Could you check a few things on this model? Use its own coordinates, in mm. A direction names the side the tool comes from. Give positions to 0.01 mm unless a question says otherwise; leave off trailing zeros. Order: outer loops, then holes, each group sorted by start corner. A loop starts at its lowest first (then second) coordinate and runs counter-clockwise, first axis right, second up. Notation, with made-up numbers: M -13,5.25 L 20,5.25 A7 ccw 20,17.25 Z; hole C -29,-28.75 d3. An arc over 180 degrees is marked long. Use a Markdown table: item, result. Add a question column.
Item 1: For faces 4 (the face through (-60.64, 61.395, 6.439)), 5 (the face through (32, 2, 12.7)), which set-ups out of +Z, -Z, +X, -X, +Y, -Y let a thin tool reach every point of the face, with its end or its side?
Item 2: Suppose I cut it at A-A on x = 0. Write out the boundary of the cut face in (y, z).
Item 3: Suppose I cut it at B-B on z = 8. Count the separate pieces of the cut face and the enclosed holes in it, plus the area to 3 significant figures.
Item 4: If I drill on L1, parallel to Y at x = 0, z = 6; L2, parallel to Y at x = -35, z = 5.5; L3, parallel to X at y = -47.5, z = 10, over which ranges is the centre line in solid material (lowest first)? Write a range as from..to.
Item 5: I'm going to push flat-ended pins straight in: pin 1 Ø1.5 at (y, z) = (-19, 1.5) entering from -X; pin 2 Ø1.5 at (y, z) = (-116, 10) entering from +X; pin 3 Ø1.5 at (x, z) = (-111, 1.5) entering from +Y. Where does each tip first touch, or does it pass through?
Item 6: If we mould it in two halves opening along Y, with no side actions, what happens to faces 1 (the face through (-125.41, -86.59, 6.26)), 2 (the face through (135.976, 42.876, 6.261)), 3 (the face through (-25.249, 140.333, 6.261))? For each: released by +Y, released by -Y, zero draft, split by the parting line, or undercut.
from build123d import *

# Parameters (mm, degrees)
F0_R     = 25.4
F1_DEPTH = 12.7
F3_DEPTH = 25.4


with BuildPart() as f1:
    # F0 (on Top) → F1 (new body)
    with BuildSketch(Plane.XY):
        with BuildLine():
            ThreePointArc((152.210637, -7.594865), (152.352652, -3.798613), (152.4, 0))
            ThreePointArc((152.4, 0), (152.380736, 2.423103), (152.322947, 4.845593))
            ThreePointArc((152.322947, 4.845593), (141.912408, 13.707712), (150.434272, 24.398564))
            ThreePointArc((150.434272, 24.398564), (149.313035, 30.518479), (147.942937, 36.587529))
            ThreePointArc((147.942937, 36.587529), (135.909535, 43.077036), (142.007699, 55.313412))
            ThreePointArc((142.007699, 55.313412), (139.631639, 61.063618), (137.022854, 66.712049))
            ThreePointArc((137.022854, 66.712049), (123.898547, 70.542066), (127.30343, 83.783034))
            ThreePointArc((127.30343, 83.783034), (123.777584, 88.909334), (120.045438, 93.887448))
            ThreePointArc((120.045438, 93.887448), (106.410408, 94.888661), (106.971492, 108.548883))
            ThreePointArc((106.971492, 108.548883), (102.451727, 112.824659), (97.761205, 116.912389))
            ThreePointArc((97.761205, 116.912389), (84.218213, 115.040539), (81.910694, 128.51614))
            ThreePointArc((81.910694, 128.51614), (76.596814, 131.752374), (71.155269, 134.769016))
            ThreePointArc((71.155269, 134.769016), (58.303006, 130.10685), (53.228892, 142.802119))
            ThreePointArc((53.228892, 142.802119), (47.355806, 144.855748), (41.403792, 146.667945))
            ThreePointArc((41.403792, 146.667945), (29.810413, 139.421563), (22.194015, 150.775282))
            ThreePointArc((22.194015, 150.775282), (16.021353, 151.555522), (9.821987, 152.083163))
            ThreePointArc((9.821987, 152.083163), (0, 142.572904), (-9.821987, 152.083163))
            ThreePointArc((-9.821987, 152.083163), (-13.282535, 151.820072), (-16.736195, 151.478249))
            ThreePointArc((-16.736195, 151.478249), (-16.661745, 150.783242), (-16.636886, 150.084702))
            ThreePointArc((-16.636886, 150.084702), (-25.44977, 140.310082), (-36.081733, 148.067108))
            ThreePointArc((-36.081733, 148.067108), (-42.095292, 146.470974), (-48.038691, 144.630717))
            ThreePointArc((-48.038691, 144.630717), (-47.5856, 142.959149), (-47.43299, 141.233999))
            ThreePointArc((-47.43299, 141.233999), (-55.223917, 131.620163), (-66.243396, 137.250036))
            ThreePointArc((-66.243396, 137.250036), (-71.790301, 134.431814), (-77.217553, 131.389533))
            ThreePointArc((-77.217553, 131.389533), (-76.085391, 128.872443), (-75.697812, 126.139803))
            ThreePointArc((-75.697812, 126.139803), (-82.489349, 116.793296), (-93.476655, 120.365589))
            ThreePointArc((-93.476655, 120.365589), (-98.311696, 116.449862), (-102.98288, 112.340048))
            ThreePointArc((-102.98288, 112.340048), (-100.909017, 109.179225), (-100.181858, 105.469379))
            ThreePointArc((-100.181858, 105.469379), (-106.007645, 96.493782), (-116.577616, 98.160172))
            ThreePointArc((-116.577616, 98.160172), (-120.487052, 93.320043), (-124.19567, 88.324377))
            ThreePointArc((-124.19567, 88.324377), (-120.970356, 84.782436), (-119.802768, 80.136498))
            ThreePointArc((-119.802768, 80.136498), (-124.707149, 71.631282), (-134.525062, 71.615415))
            ThreePointArc((-134.525062, 71.615415), (-137.336068, 66.064849), (-139.918176, 60.404173))
            ThreePointArc((-139.918176, 60.404173), (-135.39715, 56.791586), (-133.693165, 51.261044))
            ThreePointArc((-133.693165, 51.261044), (-137.730696, 43.320467), (-146.525595, 41.904774))
            ThreePointArc((-146.525595, 41.904774), (-148.113906, 35.889145), (-149.455356, 29.813698))
            ThreePointArc((-149.455356, 29.813698), (-143.569406, 26.473362), (-141.239, 20.119508))
            ThreePointArc((-141.239, 20.119508), (-144.473844, 12.83157), (-152.048709, 10.341661))
            ThreePointArc((-152.048709, 10.341661), (-152.344113, 4.126898), (-152.385603, -2.094742))
            ThreePointArc((-152.385603, -2.094742), (-145.146605, -4.804697), (-142.106697, -11.911447))
            ThreePointArc((-142.106697, -11.911447), (-144.611911, -18.465977), (-150.850248, -21.678624))
            ThreePointArc((-150.850248, -21.678624), (-149.839684, -27.817785), (-148.579381, -33.910582))
            ThreePointArc((-148.579381, -33.910582), (-140.082526, -35.634948), (-136.257897, -43.415835))
            ThreePointArc((-136.257897, -43.415835), (-138.114625, -49.164318), (-142.98319, -52.740568))
            ThreePointArc((-142.98319, -52.740568), (-140.711332, -58.532735), (-138.20495, -64.227345))
            ThreePointArc((-138.20495, -64.227345), (-128.627028, -64.632158), (-123.951157, -73.000952))
            ThreePointArc((-123.951157, -73.000952), (-125.24773, -77.87968), (-128.795312, -81.471023))
            ThreePointArc((-128.795312, -81.471023), (-125.362592, -86.660144), (-121.72093, -91.704827))
            ThreePointArc((-121.72093, -91.704827), (-111.314719, -90.494981), (-105.730518, -99.358934))
            ThreePointArc((-105.730518, -99.358934), (-106.561474, -103.31384), (-108.913814, -106.599911))
            ThreePointArc((-108.913814, -106.599911), (-104.471982, -110.956591), (-99.856025, -115.128338))
            ThreePointArc((-99.856025, -115.128338), (-88.941006, -112.063704), (-82.401454, -121.324583))
            ThreePointArc((-82.401454, -121.324583), (-82.866492, -124.311837), (-84.217593, -127.016365))
            ThreePointArc((-84.217593, -127.016365), (-78.963006, -130.34801), (-73.576812, -133.462402))
            ThreePointArc((-73.576812, -133.462402), (-62.526605, -128.371697), (-54.995268, -137.926869))
            ThreePointArc((-54.995268, -137.926869), (-55.198142, -139.913365), (-55.798387, -141.817841))
            ThreePointArc((-55.798387, -141.817841), (-49.963335, -143.977169), (-44.045008, -145.896529))
            ThreePointArc((-44.045008, -145.896529), (-33.272061, -138.688287), (-24.723496, -148.431858))
            ThreePointArc((-24.723496, -148.431858), (-24.770866, -149.395581), (-24.912517, -150.350013))
            ThreePointArc((-24.912517, -150.350013), (-18.754947, -151.241568), (-12.566119, -151.881048))
            ThreePointArc((-12.566119, -151.881048), (-2.574032, -142.549666), (7.074654, -152.235703))
            ThreePointArc((7.074654, -152.235703), (13.282535, -151.820072), (19.468278, -151.151401))
            ThreePointArc((19.468278, -151.151401), (27.288417, -139.93704), (38.749078, -147.39155))
            ThreePointArc((38.749078, -147.39155), (44.73284, -145.687107), (50.642046, -143.739846))
            ThreePointArc((50.642046, -143.739846), (55.944534, -131.138255), (68.710532, -136.031698))
            ThreePointArc((68.710532, -136.031698), (74.205652, -133.11379), (79.577094, -129.974021))
            ThreePointArc((79.577094, -129.974021), (82.127527, -116.542276), (95.634518, -118.658329))
            ThreePointArc((95.634518, -118.658329), (100.398075, -114.655948), (104.994299, -110.46247))
            ThreePointArc((104.994299, -110.46247), (104.67993, -96.794345), (118.330814, -96.039463))
            ThreePointArc((118.330814, -96.039463), (122.152227, -91.129542), (125.770049, -86.067734))
            ThreePointArc((125.770049, -86.067734), (122.604775, -72.767451), (135.796091, -69.175007))
            ThreePointArc((135.796091, -69.175007), (138.506429, -63.574596), (140.985916, -57.868224))
            ThreePointArc((140.985916, -57.868224), (135.109664, -45.523746), (147.258268, -39.252549))
            ThreePointArc((147.258268, -39.252549), (148.737713, -33.209225), (149.969257, -27.11055))
            ThreePointArc((149.969257, -27.11055), (141.641797, -16.267586), (152.210637, -7.594865))
        make_face()
        Circle(F0_R, mode=Mode.SUBTRACT)
    extrude(amount=F1_DEPTH)

    # F2 (on face) → F3 (cut)
    with BuildSketch(Plane.XY.offset(12.7)):
        with BuildLine():
            ThreePointArc((-43.530755, 9.495775), (-38.58526, 22.27721), (-29.98896, 32.950852))
            Line((-29.98896, 32.950852), (-92.160495, 90.647766))
            ThreePointArc((-92.160495, 90.647766), (-111.950573, 64.634693), (-124.583516, 34.489447))
            Line((-124.583516, 34.489447), (-43.530755, 9.495775))
        make_face()
        with BuildLine():
            Line((13.541795, 42.446627), (32.423021, 125.137213))
            ThreePointArc((32.423021, 125.137213), (0, 129.269387), (-32.423021, 125.137213))
            Line((-32.423021, 125.137213), (-13.541795, 42.446627))
            ThreePointArc((-13.541795, 42.446627), (0, 44.554421), (13.541795, 42.446627))
        make_face()
        with BuildLine():
            ThreePointArc((29.98896, 32.950852), (38.58526, 22.27721), (43.530755, 9.495775))
            Line((43.530755, 9.495775), (124.583516, 34.489447))
            ThreePointArc((124.583516, 34.489447), (111.950573, 64.634693), (92.160495, 90.647766))
            Line((92.160495, 90.647766), (29.98896, 32.950852))
        make_face()
        with BuildLine():
            ThreePointArc((43.530755, -9.495775), (38.58526, -22.27721), (29.98896, -32.950852))
            Line((29.98896, -32.950852), (92.160495, -90.647766))
            ThreePointArc((92.160495, -90.647766), (111.950573, -64.634693), (124.583516, -34.489447))
            Line((124.583516, -34.489447), (43.530755, -9.495775))
        make_face()
        with BuildLine():
            ThreePointArc((13.541795, -42.446627), (0, -44.554421), (-13.541795, -42.446627))
            Line((-13.541795, -42.446627), (-32.423021, -125.137213))
            ThreePointArc((-32.423021, -125.137213), (0, -129.269387), (32.423021, -125.137213))
            Line((32.423021, -125.137213), (13.541795, -42.446627))
        make_face()
        with BuildLine():
            ThreePointArc((-29.98896, -32.950852), (-38.58526, -22.27721), (-43.530755, -9.495775))
            Line((-43.530755, -9.495775), (-124.583516, -34.489447))
            ThreePointArc((-124.583516, -34.489447), (-111.950573, -64.634693), (-92.160495, -90.647766))
            Line((-92.160495, -90.647766), (-29.98896, -32.950852))
        make_face()
    extrude(amount=-F3_DEPTH, mode=Mode.SUBTRACT)


solid = f1.part
Findings below:
| question | item | result |
|---|---|---|
| 1 | face 4 | +Z, -Z |
| 1 | face 5 | +Z, +X, -X, +Y, -Y |
| 2 | outline | M -142.94,0 L -129.27,0 L -129.27,12.7 L -142.94,12.7 Z; M -44.55,0 L -25.4,0 L -25.4,12.7 L -44.55,12.7 Z; M 25.4,0 L 44.55,0 L 44.55,12.7 L 25.4,12.7 Z; M 129.27,0 L 142.57,0 L 142.57,12.7 L 129.27,12.7 Z |
| 3 | separate pieces | 1 |
| 3 | enclosed holes | 7 |
| 3 | area | 42,800 mm^2 |
| 4 | L1 | y = -142.94..-129.27, -44.55..-25.4, 25.4..44.55, 129.27..142.57 |
| 4 | L2 | y = -138.62..-37.6, -27.57..27.57, 37.6..145.22 |
| 4 | L3 | x = -137.15..-120.23, -45.67..-14.7, 14.7..45.67, 120.23..134.66 |
| 5 | pin 1 | stops at x = -146.01 |
| 5 | pin 2 | stops at x = 99.72 |
| 5 | pin 3 | stops at y = 95.8 |
| 6 | face 1 | released by -Y |
| 6 | face 2 | undercut |
| 6 | face 3 | released by +Y |
